The model under review builds one solid part; all positions refer to its coordinate system, in mm. Face numbers are marked on the shaded views. A direction names the side the tool comes from. Coordinates: 2 decimals unless noted, no trailing zeros. Order: outer loops, then holes, each group sorted by start corner. A loop starts at its lowest first (then second) coordinate and runs counter-clockwise, first axis right, second up.
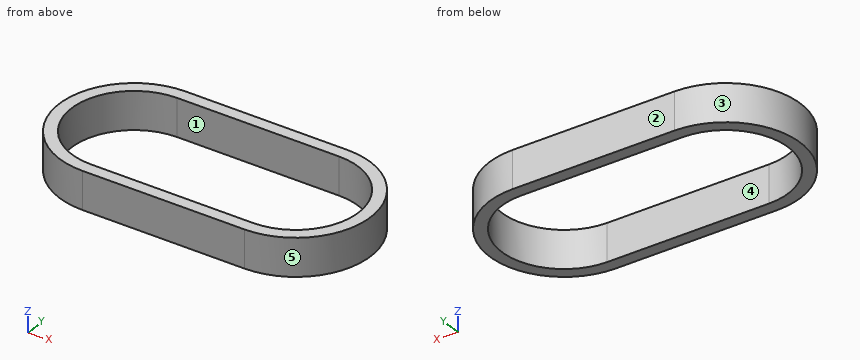
```python
from build123d import *

# Parameters (mm, degrees)
BOSS_EXTRU_1_DEPTH = 3


with BuildPart() as part:
    # Esquisse1 → Boss.-Extru.1 (new, symmetric)
    # profile 1 of 2: a face of its own
    with BuildSketch(Plane.XY):
        with BuildLine():
            Line((0, 11.86), (25.5, 11.86))
            ThreePointArc((25.5, 11.86), (37.36, 0), (25.5, -11.86))
            Line((25.5, -11.86), (0, -11.86))
            ThreePointArc((0, -11.86), (-11.86, 0), (0, 11.86))
        make_face()
        with BuildLine():
            ThreePointArc((25.5, -11.46), (36.96, 0), (25.5, 11.46))
            Line((25.5, 11.46), (0, 11.46))
            ThreePointArc((0, 11.46), (-11.46, 0), (0, -11.46))
            Line((0, -11.46), (25.5, -11.46))
        make_face(mode=Mode.SUBTRACT)
    # profile 2 of 2: a face of its own
    with BuildSketch(Plane.XY):
        with BuildLine():
            Line((0, -11.46), (25.5, -11.46))
            ThreePointArc((25.5, -11.46), (36.96, 0), (25.5, 11.46))
            Line((25.5, 11.46), (0, 11.46))
            ThreePointArc((0, 11.46), (-11.46, 0), (0, -11.46))
        make_face()
        with BuildLine():
            ThreePointArc((0, 9.92), (-9.92, 0), (0, -9.92))
            Line((0, -9.92), (25.5, -9.92))
            ThreePointArc((25.5, -9.92), (35.42, 0), (25.5, 9.92))
            Line((25.5, 9.92), (0, 9.92))
        make_face(mode=Mode.SUBTRACT)
    extrude(amount=BOSS_EXTRU_1_DEPTH, both=True)


solid = part.part
```
(1) For pin 1 Ø2 at (y, z) = (1, 0) entering from -X; pin 2 Ø1 at (y, z) = (-1, 2) entering from +X; pin 3 Ø1.5 at (y, z) = (6, -1) entering from -X; pin 4 Ø10 at (x, y) = (15, 4.5) entering from -Z, all flat-tipped, find the tip position at first contact; note any pin that passes through.
A:
pin 1: stops at x = -11.86
pin 2: stops at x = 37.35
pin 3: stops at x = -10.63
pin 4: passes through
(2) We need section A-A, the plane x = 4.5. Write out the cut boundary in (y, z), and give its area (3 significant figures).
A:
outline: (-11.86, -3) - (-9.92, -3) - (-9.92, 3) - (-11.86, 3) - close; (9.92, -3) - (11.86, -3) - (11.86, 3) - (9.92, 3) - close
area: 23.3 mm2
(3) Machinability: for the marked faces 1 and 2, which of the approach directions +Z, -Z, +X, -X, +Y, -Y give a long, thin tool a straight path to every point of the face, cutting with its end or side? Answer none if there is none.
A:
face 1: +Z, -Z
face 2: +Z, -Z, +X, -X, +Y
(4) We need section B-B, the plane y = 0. Write out the cut boundary in (x, z), and give its area (3 significant figures).
A:
outline: (-11.86, -3) - (-9.92, -3) - (-9.92, 3) - (-11.86, 3) - close; (35.42, -3) - (37.36, -3) - (37.36, 3) - (35.42, 3) - close
area: 23.3 mm2
(5) We need section C-C, the plane z = -1.4. Write out the cut boundary in (x, y), and give its area (3 significant figures).
A:
outline: (0, -11.86) - (25.5, -11.86) arc R11.86 ccw to (25.5, 11.86) - (0, 11.86) arc R11.86 ccw to start; hole (0, -9.92) - (25.5, -9.92) arc R9.92 ccw to (25.5, 9.92) - (0, 9.92) arc R9.92 ccw to start
area: 232 mm2
(6) Wall thickness on probe 1 along Y at (x, z) = (9, -2.45); probe 2 along Y at (x, z) = (27.5, -1.55); probe 3 along X at (y, z) = (3.25, 2.4): over which ranges is each line inside the solid? List them lowest first.
A:
probe 1: y = -11.86 to -9.92, 9.92 to 11.86
probe 2: y = -11.69 to -9.72, 9.72 to 11.69
probe 3: x = -11.41 to -9.37, 34.87 to 36.91
(7) Draft analysis for pull direction X (two halves, no side actions). For the marked faces 3, 4 and 5, state which applies: released by +X, released by -X, zero draft, split by the parting line, or undercut.
A:
face 3: released by -X
face 4: undercut
face 5: released by +X
